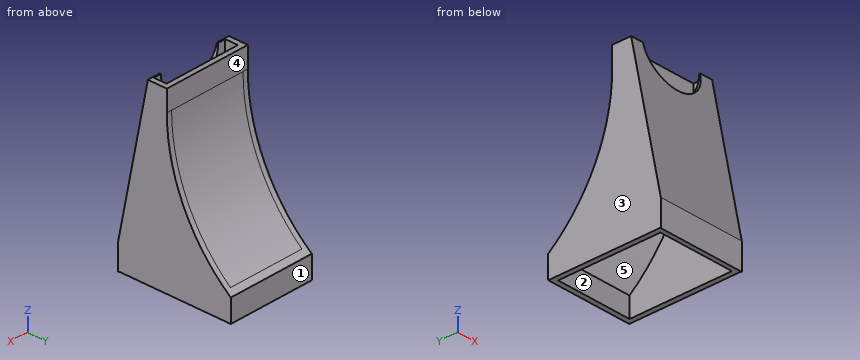
```python
from build123d import *

# Parameters (mm, degrees)
SKETCH1_W           = 17
SKETCH1_H           = 22
SKETCH1_W_2         = 15
SKETCH1_H_2         = 20
BOSS_EXTRUDE1_DEPTH = 30
SKETCH2_R           = 32.5
CUT_EXTRUDE1_DEPTH  = 37.193922142
BOSS_EXTRUDE2_REACH = 38.194
CUT_EXTRUDE2_DEPTH  = 37.193922142
BOSS_EXTRUDE3_START = -17
BOSS_EXTRUDE3_DEPTH = 17
SKETCH6_W           = 17
SKETCH6_H           = 4.5
SKETCH6_W_2         = 15
SKETCH6_H_2         = 2.480196097
BOSS_EXTRUDE4_DEPTH = 4
CUT_EXTRUDE3_DEPTH  = 40.572717875
CUT_EXTRUDE4_REACH  = 41.807
SKETCH8_R           = 6


with BuildPart() as part:
    # Sketch1 → Boss-Extrude1 (new body)
    with BuildSketch(Plane.XY):
        Rectangle(SKETCH1_W, SKETCH1_H)
        Rectangle(SKETCH1_W_2, SKETCH1_H_2, mode=Mode.SUBTRACT)
    extrude(amount=BOSS_EXTRUDE1_DEPTH)

    # Sketch2 → Cut-Extrude1 (cut, through all)
    with BuildSketch(Plane(origin=(8.5, 0, 0), x_dir=(0, 0, -1), z_dir=(1, 0, 0))):
        with Locations((-30, 31)):
            Circle(SKETCH2_R)
    extrude(amount=-CUT_EXTRUDE1_DEPTH, mode=Mode.SUBTRACT)

    # Sketch3 → Boss-Extrude2 (add, up to next)
    with BuildSketch(Plane(origin=(8.5, 0, 0), x_dir=(0, 0, -1), z_dir=(1, 0, 0)), mode=Mode.PRIVATE) as boss_extrude2_sk1:
        with BuildLine():
            Line((-30, -1.5), (-30, -2.5))
            ThreePointArc((-30, -2.5), (-14.962546758, 1.064653), (-3.125290699, 11))
            Line((-3.125290699, 11), (-4.382623085, 11))
            ThreePointArc((-4.382623085, 11), (-15.747807186, 1.791696386), (-30, -1.5))
        make_face()
    boss_extrude2_tool1 = extrude(boss_extrude2_sk1.sketch, amount=-BOSS_EXTRUDE2_REACH, mode=Mode.PRIVATE) - part.part
    add(boss_extrude2_tool1.solids().sort_by_distance((8.5, 1.521408, 15.61592))[0])

    # Sketch4 → Cut-Extrude2 (cut, through all)
    with BuildSketch(Plane.ZY.offset(8.5)):
        Polygon((5, -11), (30, -6), (30, -11), align=None)
    extrude(amount=-CUT_EXTRUDE2_DEPTH, mode=Mode.SUBTRACT)

    # Sketch5 → Boss-Extrude3 (add)
    with BuildSketch(Plane.ZY.offset(8.5).offset(BOSS_EXTRUDE3_START)):
        Polygon((5, -11), (30, -6), (30, -4.980196097), (-0.099019514, -11), align=None)
    extrude(amount=BOSS_EXTRUDE3_DEPTH)

    # Sketch6 → Boss-Extrude4 (add)
    with BuildSketch(Plane.XY.offset(30)):
        with Locations((0, -3.75)):
            Rectangle(SKETCH6_W, SKETCH6_H)
        with Locations((0, -3.740098049)):
            Rectangle(SKETCH6_W_2, SKETCH6_H_2, mode=Mode.SUBTRACT)
    extrude(amount=BOSS_EXTRUDE4_DEPTH)

    # Sketch7 → Cut-Extrude3 (cut, through all)
    with BuildSketch(Plane.ZY.offset(8.5)):
        Polygon((24, -7.2), (34, -5.2), (34, -7.2), align=None)
    extrude(amount=-CUT_EXTRUDE3_DEPTH, mode=Mode.SUBTRACT)

    # Sketch8 → Cut-Extrude4 (cut, up to next)
    with BuildSketch(Plane(origin=(0, -11.538461538, 2.307692308), x_dir=(1, 0, 0), z_dir=(0, -0.9805806756909202, 0.19611613513818413)), mode=Mode.PRIVATE) as cut_extrude4_sk1:
        with Locations((0, 32.319939071)):
            Circle(SKETCH8_R)
    cut_extrude4_tool1 = extrude(cut_extrude4_sk1.sketch, amount=-CUT_EXTRUDE4_REACH, mode=Mode.PRIVATE) & part.part
    add(cut_extrude4_tool1.solids().sort_by_distance((0, -5.2, 34))[0], mode=Mode.SUBTRACT)


solid = part.part
```
Check sheet for the modelled part. Datum: model origin and axes. Units: mm. Face numbers are marked on the shaded views. A direction names the side the tool comes from. Round coordinates to 2 decimals unless told otherwise and drop trailing zeros. Loops run counter-clockwise (first coordinate to the right, second up) from the corner with the lowest first, then second, coordinate; pieces in that order, holes last. Notation, with made-up numbers: (0.5, -6) - (35.5, -6) arc R21 ccw to (35.5, -2) - close; hole circle Ø3 at (14.5, 3). An arc over 180 degrees is marked (long way). Answer as a JSON object with one key per item and string values. Group by question number.
Q1. Sectioned sample at D-D, the plane y = 5.5. Enter the section's corners in (x, z), plus the area to 3 significant figures.
Q2. Scan lines: line 1 along X through (y, z) = (4.25, 5.5); line 2 along Y through (x, z) = (6.75, 25); line 3 along Y through (x, z) = (5.5, 13). Record each from-to range of solid material in increasing order. Write a range as [from, to].
Q3. Set-up check for the marked faces 1 and 2: record each of +Z, -Z, +X, -X, +Y, -Y from which the full face is reachable in a straight line by a thin tool's end or side.
Q4. Mould release check, pull along X, two halves, no side actions. Record for the marked faces 3, 4 and 5: released by +X, released by -X, zero draft, split by the parting line, or undercut.
Q5. Sectioned sample at B-B, the plane x = -2.75. Enter the section's corners in (y, z).
Q6. Sectioned sample at A-A, the plane y = -3.75. Enter the section's corners in (x, z), plus the area to 3 significant figures.
Q7. Sectioned sample at C-C, the plane z = 10. Enter the section's corners in (x, y).
Q8. Gauge pin test, flat ends, axial feed: P1, Ø1.5, axis at x = -5.5, z = 32, coming from the +Y side; P2, Ø8, axis at x = 4, z = 23, coming from the -Y side; P3, Ø8, axis at x = 5, y = 6, coming from the -Z side. Record the tip position at first contact, or that the pin passes through.
Solution:
{
 "1": {"outline": "(-8.5, 0) - (-7.5, 0) - (-7.5, 8.27) - (7.5, 8.27) - (7.5, 0) - (8.5, 0) - (8.5, 9.85) - (-8.5, 9.85) - close", "area": "43.3 mm²"},
 "2": {"line 1": "x = [-8.5, -7.5], [7.5, 8.5]", "line 2": "y = [-7, -5.98], [-2.12, -1.11]", "line 3": "y = [-9.4, -8.38], [2.13, 3.3]"},
 "3": {"face 1": "+Z, -Z, +X, -X, +Y", "face 2": "-Z"},
 "4": {"face 3": "released by -X", "face 4": "zero draft", "face 5": "undercut"},
 "5": {"outline": "(-11, -0.1) - (-10.98, 0) - (-10, 0) - (-10, 4.9) - (-5.27, 28.57) - (-6.25, 28.77) - (-11, 5) - close; (-2.5, 30) arc R33.5 ccw to (10, 3.9) - (10, 0) - (11, 0) - (11, 4.38) arc R32.5 cw to (-1.5, 30) - (-1.5, 34) - (-2.5, 34) - close"},
 "6": {"outline": "(-8.5, 0) - (-7.5, 0) - (-7.5, 34) - (-8.5, 34) - close; (7.5, 0) - (8.5, 0) - (8.5, 34) - (7.5, 34) - close", "area": "68.0 mm²"},
 "7": {"outline": "(-8.5, -10) - (8.5, -10) - (8.5, 5.38) - (-8.5, 5.38) - close; hole (-7.5, -8.98) - (7.5, -8.98) - (7.5, 4.13) - (-7.5, 4.13) - close"},
 "8": {"P1": "stops at y = -1.5", "P2": "stops at y = -8.2", "P3": "stops at z = 0"}
}
